The listing builds one solid part. Answer for the finished solid, in the listing's coordinates (mm). Face numbers are marked on the shaded views. A direction names the side the tool comes from. Coordinates: 2 decimals unless noted, no trailing zeros. Order: outer loops, then holes, each group sorted by start corner. A loop starts at its lowest first (then second) coordinate and runs counter-clockwise, first axis right, second up.
```python
from build123d import *

# Parameters (mm, degrees)
ENL_V_MAT_EXTRU_1_DEPTH      = 38.559086783
R_P_TITION_CIRCULAIRE1_COUNT = 3
ESQUISSE5_R                  = 0.7
BOSS_EXTRU_1_DEPTH           = 25


with BuildPart() as part:
    # Esquisse1 → R_volution1 (revolve)
    with BuildSketch(Plane.XY, mode=Mode.PRIVATE) as r_volution1_sk:
        Polygon((0, 0), (50, 0), (50, 1), (47, 1), (47, 2.95), (43.6, 2.95), (43.6, 8.2), (26.6, 8.2), (26.6, 17), (10.6, 17), (4.6, 18.75), (4.6, 5.75), (0, 3.370541895), align=None)
    revolve(r_volution1_sk.sketch.rotate(Axis((0, 0, 0), (1, 0, 0)), 90), axis=Axis((0, 0, 0), (1, 0, 0)))

    # Esquisse4 → Enl_v. mat.-Extru.1 (cut, through all)
    with BuildSketch(Plane(origin=(26.6, 0, 0), x_dir=(0, 0, -1), z_dir=(1, 0, 0))):
        with BuildLine():
            Line((-0.7, 15.984680166), (-0.7, 9.173330911))
            ThreePointArc((-0.7, 9.173330911), (-7.967433715, 4.6), (-8.294337606, -3.980447673))
            Line((-8.294337606, -3.980447673), (-14.193139095, -7.3861223))
            ThreePointArc((-14.193139095, -7.3861223), (-13.856406461, 8), (-0.7, 15.984680166))
        make_face()
    enl_v_mat_extru_1 = extrude(amount=-ENL_V_MAT_EXTRU_1_DEPTH, mode=Mode.SUBTRACT)

    # R_p_tition circulaire1: Enl_v. mat.-Extru.1 ×3 about axis
    r_p_tition_circulaire1_axis = Axis((0, 0, 0), (1, 0, 0))
    for i in range(1, R_P_TITION_CIRCULAIRE1_COUNT):
        add(enl_v_mat_extru_1.rotate(r_p_tition_circulaire1_axis, i * 360 / R_P_TITION_CIRCULAIRE1_COUNT), mode=Mode.SUBTRACT)

    # Esquisse5 → Boss.-Extru.1 (add)
    with BuildSketch(Plane(origin=(0, 0, 0), x_dir=(1, 0, 0), z_dir=(0, 1, 0))):
        with Locations(Location((27.361357126, 0, 0), (0, 0, 90))):
            Circle(ESQUISSE5_R)
        with Locations(Location((27.361357126, 2.007154896, 0), (0, 0, 90))):
            Circle(ESQUISSE5_R)
        with Locations(Location((27.361357126, -2.007154896, 0), (0, 0, 90))):
            Circle(ESQUISSE5_R)
    extrude(amount=BOSS_EXTRU_1_DEPTH)


solid = part.part
```
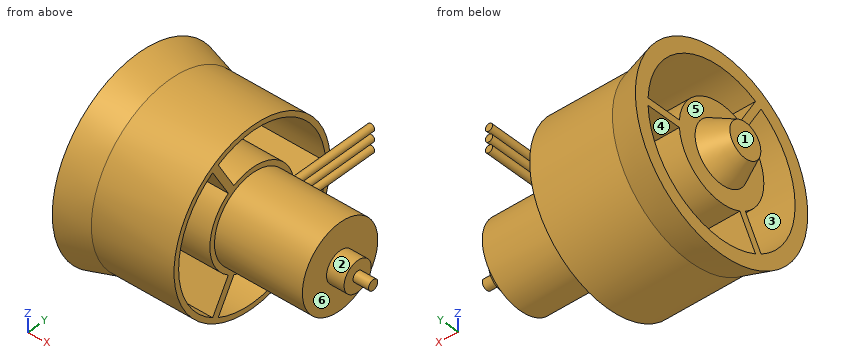
1) For the marked faces 4, 5 and 6, determine the directions among +Z, -Z, +X, -X, +Y, -Y from which every point of the face is accessible in a straight line to the end or side of a thin tool.
2) Each of these flat-tipped pins is pushed along its axis until it touches: P1, Ø4, axis at x = 25.5, y = -4.5, coming from the +Z side; P2, Ø5.5, axis at x = 15, y = 13.5, coming from the -Z side; P3, Ø5, axis at x = 8, z = -6, coming from the +Y side; P4, Ø6.5, axis at y = 0.5, z = 1, coming from the +X side. Where does it stop, or does it pass through?
3) Straight lines are drawn through the part: probe 1 along Y at (x, z) = (5, -4.5); probe 2 along Y at (x, z) = (23, 5); probe 3 along Z at (x, y) = (10, -0.5). For each, find the intervals that lie inside material, in ascending order.
4) A cutting plane is placed at D-D, the plane z = -12.5. Count the separate pieces of the cut face and the enclosed holes in it, plus the area to 3 significant figures.
5) A cutting plane is placed at C-C, the plane x = 45.5. Write down the section's boundary in (y, z), plus the area to 3 significant figures.
6) A cutting plane is placed at A-A, the plane x = 17. Write down the section's boundary in (y, z).
7) The mould has two halves that part along Y. Classify the marked faces 1, 2 and 3: released by +Y, released by -Y, zero draft, split by the parting line, or undercut.
Working result:
1. face 4: +X, -X
1. face 5: -X
1. face 6: +X
2. P1: stops at z = 16.82
2. P2: stops at z = -13.17
2. P3: stops at y = 17.78
2. P4: stops at x = 50
3. probe 1: y = -18.08 to -15.35, -8.02 to 8.02, 15.35 to 18.08
3. probe 2: y = -16.25 to -15.2, -7.72 to 7.72, 15.2 to 16.25
3. probe 3: z = -17.17 to -15.99, -9.19 to 9.19, 15.99 to 17.17
4. separate pieces: 3
4. enclosed holes: 0
4. area: 118 mm2
5. outline: circle Ø5.9 at (0, 0)
5. area: 27.3 mm2
6. outline: circle Ø34 at (0, 0); hole (-8.6, -13.49) - (-5.19, -7.59) arc R9.2 cw to (-5.19, 7.59) - (-8.6, 13.49) arc R16 ccw to start; hole (-7.39, -14.19) arc R16 ccw to (15.98, -0.7) - (9.17, -0.7) arc R9.2 cw to (-3.98, -8.29) - close; hole (-7.39, 14.19) - (-3.98, 8.29) arc R9.2 cw to (9.17, 0.7) - (15.98, 0.7) arc R16 ccw to start
7. face 1: zero draft
7. face 2: split by the parting line
7. face 3: undercut
